CAD build for the part. Positions are in the model's coordinates, mm. Face numbers are marked on the shaded views. Round coordinates to 2 decimals unless told otherwise and drop trailing zeros. Order: outer loops, then holes, each group sorted by start corner. A loop starts at its lowest first (then second) coordinate and runs counter-clockwise, first axis right, second up. Notation, with made-up numbers: M 22.25,-38 L 47.25,-38 A29 cw 47.25,-18 Z; hole C 6.5,-27.5 d8. An arc over 180 degrees is marked long. Answer as a JSON object with one key per item and string values.
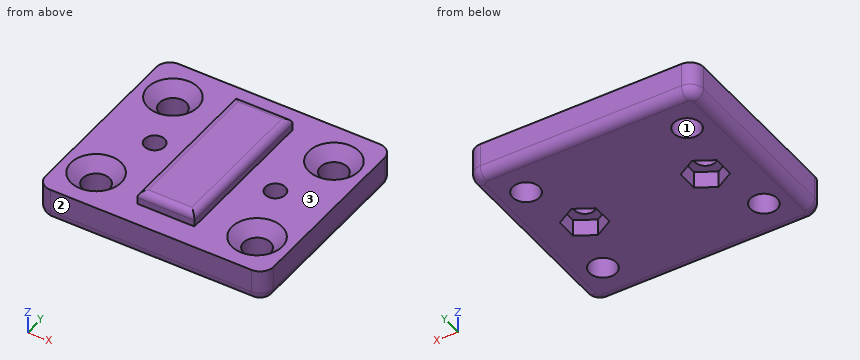
```python
from build123d import *

# Parameters (mm, degrees)
F0_W      = 34
F0_H      = 30
F0_R      = 2
F1_DEPTH  = 5
F2_R      = 1.5
F3_DEPTH  = 5
F4_SIZE   = 1.75
F5_R      = 1.5
F6_DEPTH  = 2.5
F8_R      = 2
F9_R      = 1.5
F10_W     = 8.5
F10_H     = 23
F11_DEPTH = 2
F12_R     = 1


with BuildPart() as f1:
    # F0 (on Top) → F1 (new body)
    with BuildSketch(Plane.XY):
        Rectangle(F0_W, F0_H)
        with Locations((-12, -9)):
            Circle(F0_R, mode=Mode.SUBTRACT)
        with Locations((12, -9)):
            Circle(F0_R, mode=Mode.SUBTRACT)
        with Locations((-12, 9)):
            Circle(F0_R, mode=Mode.SUBTRACT)
        with Locations((12, 9)):
            Circle(F0_R, mode=Mode.SUBTRACT)
    extrude(amount=F1_DEPTH)

    # F2 (on face) → F3 (cut, through all)
    with BuildSketch(Plane.XY.offset(5)):
        with Locations((9, 0)):
            Circle(F2_R)
        with Locations((-9, 0)):
            Circle(F2_R)
    extrude(amount=-F3_DEPTH, mode=Mode.SUBTRACT)

    # F4
    f4_edges = [f1.edges().sort_by_distance(p)[0] for p in [
        (-14, -9, 5),
        (-14, 9, 5),
        (10, 9, 5),
        (10, -9, 5),
    ]]
    chamfer(f4_edges, length=F4_SIZE)

    # F5 (on face) → F6 (cut)
    with BuildSketch(Plane(origin=(0, 0, 0), x_dir=(1, 0, 0), z_dir=(0, 0, -1))):
        Polygon((-6.3, -1.558846), (-6.3, 1.558846), (-9, 3.117691), (-11.7, 1.558846), (-11.7, -1.558846), (-9, -3.117691), align=None)
        with Locations((-9, 0)):
            Circle(F5_R, mode=Mode.SUBTRACT)
        Polygon((6.3, 1.558846), (6.3, -1.558846), (9, -3.117691), (11.7, -1.558846), (11.7, 1.558846), (9, 3.117691), align=None)
        with Locations((9, 0)):
            Circle(F5_R, mode=Mode.SUBTRACT)
    extrude(amount=-F6_DEPTH, mode=Mode.SUBTRACT)

    # F8
    f8_edges = [f1.edges().sort_by_distance(p)[0] for p in [
        (17, -15, 2.5),
        (17, 15, 2.5),
        (-17, -15, 2.5),
        (-17, 15, 2.5),
    ]]
    fillet(f8_edges, radius=F8_R)

    # F9
    f9_edges = [f1.edges().sort_by_distance(p)[0] for p in [
        (0, -15, 0),
    ]]
    fillet(f9_edges, radius=F9_R)

    # F10 (on face) → F11 (join)
    with BuildSketch(Plane.XY.offset(5)):
        Rectangle(F10_W, F10_H)
    extrude(amount=F11_DEPTH)

    # F12
    f12_edges = [f1.edges().sort_by_distance(p)[0] for p in [
        (0, -11.5, 7),
        (4.25, 0, 7),
        (-4.25, 0, 7),
        (0, 11.5, 7),
    ]]
    fillet(f12_edges, radius=F12_R)


solid = f1.part
```
Item 1: Drop flat-ended pins along their axis: pin 1 Ø0.5 at (x, z) = (1, 5.5) entering from +Y; pin 2 Ø1.5 at (x, y) = (9.5, -10.5) entering from +Z; pin 3 Ø3.5 at (x, y) = (9, 0) entering from +Z; pin 4 Ø2.5 at (x, y) = (12, -9) entering from +Z. Give the stop position or say it passes through.
Worked answers:
{"pin 1": "stops at y = 11.5", "pin 2": "stops at z = 4.92", "pin 3": "stops at z = 5", "pin 4": "passes through"}
Item 2: Saw through at B-B on x = -2.5. List the corners of the cut face in (y, z), and give its area (3 significant figures).
Worked answers:
{"outline": "M -15,1.5 A1.5 ccw -13.5,0 L 13.5,0 A1.5 ccw 15,1.5 L 15,5 L 11.5,5 L 11.5,6 A1 ccw 10.5,7 L -10.5,7 A1 ccw -11.5,6 L -11.5,5 L -15,5 Z", "area": "195 mm2"}
Item 3: Two-plate mould, pull along Y, no slides. Class the marked faces 1, 2 and 3: released by +Y, released by -Y, zero draft, split by the parting line, or undercut.
Worked answers:
{"face 1": "undercut", "face 2": "released by -Y", "face 3": "zero draft"}
Item 4: Wall check: line 1 along Y through (x, z) = (-12, 2.25); line 2 along X through (y, z) = (0, 3.65); line 3 along Y through (x, z) = (-9, 3.15). Give the ranges that are in metal, low to high. Write a range as [from, to].
Worked answers:
{"line 1": "y = [-15, -11], [-7, 7], [11, 15]", "line 2": "x = [-17, -10.5], [-7.5, 7.5], [10.5, 17]", "line 3": "y = [-15, -1.5], [1.5, 15]"}
Item 5: Saw through at A-A on y = 0. List the corners of the cut face in (x, z), and give its area (3 significant figures).
Worked answers:
{"outline": "M -17,1.5 A1.5 ccw -15.5,0 L -11.7,0 L -11.7,2.5 L -10.5,2.5 L -10.5,5 L -17,5 Z; M -7.5,2.5 L -6.3,2.5 L -6.3,0 L 6.3,0 L 6.3,2.5 L 7.5,2.5 L 7.5,5 L 4.25,5 L 4.25,6 A1 ccw 3.25,7 L -3.25,7 A1 ccw -4.25,6 L -4.25,5 L -7.5,5 Z; M 10.5,2.5 L 11.7,2.5 L 11.7,0 L 15.5,0 A1.5 ccw 17,1.5 L 17,5 L 10.5,5 Z", "area": "144 mm2"}
Item 6: Saw through at C-C on y = 9. List the corners of the cut face in (x, z), and give its area (3 significant figures).
Worked answers:
{"outline": "M -17,1.5 A1.5 ccw -15.5,0 L -14,0 L -14,3.25 L -15.75,5 L -17,5 Z; M -10,0 L 10,0 L 10,3.25 L 8.25,5 L 4.25,5 L 4.25,6 A1 ccw 3.25,7 L -3.25,7 A1 ccw -4.25,6 L -4.25,5 L -8.25,5 L -10,3.25 Z; M 14,0 L 15.5,0 A1.5 ccw 17,1.5 L 17,5 L 15.75,5 L 14,3.25 Z", "area": "139 mm2"}
Item 7: Saw through at D-D on y = -8.5. State how many separate pieces and enclosed holes the cut face has, and give its area (3 significant figures).
Worked answers:
{"separate pieces": "3", "enclosed holes": "0", "area": "141 mm2"}
